Study the drawing (mm; zero at the part's minimum x, y, z) and answer. A direction names the side the tool comes from. Round coordinates to 2 decimals unless told otherwise and drop trailing zeros. Loops run counter-clockwise (first coordinate to the right, second up) from the corner with the lowest first, then second, coordinate; pieces in that order, holes last. Notation, with made-up numbers: (62.5, -23) -> (111.5, -23) arc R11 ccw to (111.5, -4) -> close; hole circle Ø3 at (6.25, 45.25). An arc over 180 degrees is marked (long way). Use one line per item in the form item = value.
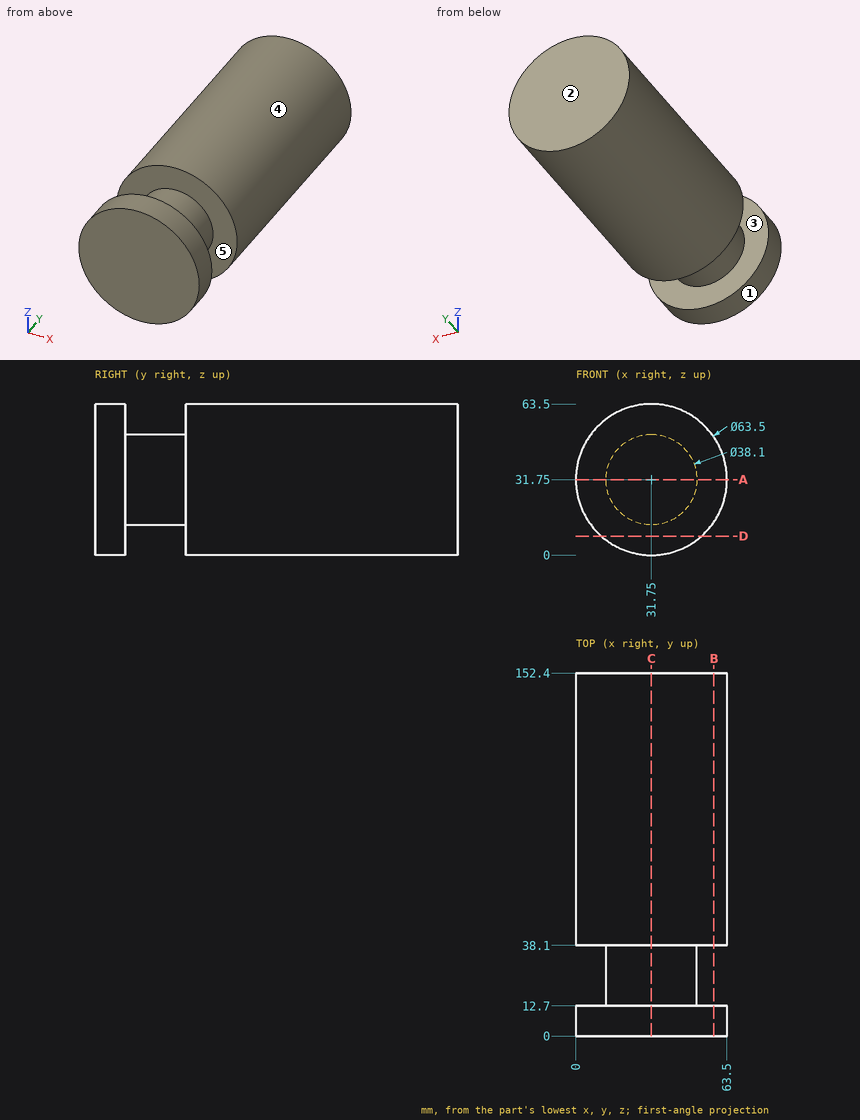
(1) For a pull along Y with two mould halves and no side action, classify the marked faces 1, 2 and 3 as +Y half, -Y half, draft (parallel to the pull), parting line (faces both ways), or undercut.
Completed:
face_1 = draft
face_2 = +Y half
face_3 = undercut
(2) For the marked faces 4 and 5, determine the directions among +Z, -Z, +X, -X, +Y, -Y from which every point of the face is accessible in a straight line to the end or side of a thin tool.
Completed:
face_4 = +Y, -Y
face_5 = none
(3) Find section C-C, the plane x = 31.75. Write down the section's boundary in (y, z), then the cut area to 3 significant figures.
Completed:
outline = (0, 0) -> (12.7, 0) -> (12.7, 12.7) -> (38.1, 12.7) -> (38.1, 0) -> (152.4, 0) -> (152.4, 63.5) -> (38.1, 63.5) -> (38.1, 50.8) -> (12.7, 50.8) -> (12.7, 63.5) -> (0, 63.5) -> close
area = 9,030 mm2
(4) Find section A-A, the plane z = 31.75. Write down the section's boundary in (x, y), then the cut area to 3 significant figures.
Completed:
outline = (0, 0) -> (63.5, 0) -> (63.5, 12.7) -> (50.8, 12.7) -> (50.8, 38.1) -> (63.5, 38.1) -> (63.5, 152.4) -> (0, 152.4) -> (0, 38.1) -> (12.7, 38.1) -> (12.7, 12.7) -> (0, 12.7) -> close
area = 9,030 mm2
(5) Given P1, Ø2, axis at x = 13, y = 123, coming from the +Z side; P2, Ø10, axis at x = 6.5, z = 14.5, coming from the -Y side; P3, Ø1.5, axis at x = 13.5, y = 106, coming from the +Z side; P4, Ø8, axis at x = 56, y = 46, coming from the -Z side, each flat-ended and moving along its own axis, determine where each tip first touches the part or whether it passes through.
Completed:
P1 = 58.07
P2 = 0
P3 = 58.24
P4 = 7.3
(6) Consider L1, parallel to Y at x = 30.5, z = 7; L2, parallel to X at y = 107.5, z = 32.5; L3, parallel to X at y = 105.5, z = 48. Determine where each line is inside the solid, lowest interval first.
Completed:
L1 = 0 to 12.7, 38.1 to 152.4
L2 = 0.01 to 63.49
L3 = 4.47 to 59.03
(7) Find section D-D, the plane z = 8. Write down the section's boundary in (x, y).
Completed:
outline = (10.68, 0) -> (52.82, 0) -> (52.82, 12.7) -> (10.68, 12.7) -> close; (10.68, 38.1) -> (52.82, 38.1) -> (52.82, 152.4) -> (10.68, 152.4) -> close
(8) Find section B-B, the plane x = 58. Write down the section's boundary in (y, z), then the cut area to 3 significant figures.
Completed:
outline = (0, 13.89) -> (12.7, 13.89) -> (12.7, 49.61) -> (0, 49.61) -> close; (38.1, 13.89) -> (152.4, 13.89) -> (152.4, 49.61) -> (38.1, 49.61) -> close
area = 4,540 mm2
